The model under review builds one solid part; all positions refer to its coordinate system, in mm. A direction names the side the tool comes from. Coordinates: 2 decimals unless noted, no trailing zeros. Write each loop counter-clockwise with the first axis right and the second up, starting at its lowest first coordinate (ties: lowest second). Pieces come first, ordered by that corner, then holes. Notation, with made-up numbers: (58, 47) - (70, 47) arc R21 cw to (70, 86) - close; hole circle Ø5 at (13.25, 28.5). An arc over 180 degrees is marked (long way). Put each result on its own line as item: value. Start each with the question number.
Item 1: For pin 1 (2.5 mm diameter, centred on y = 47.5, z = -42.5, fed in from +X); pin 2 (1 mm diameter, centred on y = 2, z = -11.5, fed in from +X); pin 3 (12.5 mm diameter, centred on x = 39.41, y = 63.5, fed in from -Z); pin 4 (1.5 mm diameter, centred on y = 15, z = 37, fed in from +X), all flat-tipped, find the tip position at first contact; note any pin that passes through.
Item 2: Machinability: for faces 4 (the face through (-47, 2, 21.902)), 5 (the face through (17.18, 2, 13)), 6 (the face through (-47, 75, -0.323)), 7 (the face through (-4.796, 28.121, 67.961)), 8 (the face through (-38, 73.025, -12)), which of the approach directions +Z, -Z, +X, -X, +Y, -Y give a long, thin tool a straight path to every point of the face, cutting with its end or side? Answer none if there is none.
Item 3: Consider section D-D on y = 68.5. Give the boundary of the cut face in (x, z), then the cut area to 3 significant figures.
Item 4: Consider section B-B on x = 1. State how many separate pieces and enclosed holes the cut face has, then the cut area to 3 significant figures.
Item 5: Consider section A-A on z = 6.5. Give the boundary of the cut face in (x, y) (1 decimal).
Item 6: To check wall thickness, follow L1, parallel to Z at x = 34, y = 69.5; L2, parallel to Y at x = 6, z = -34 (3 decimals); L3, parallel to X at y = 24.5, z = 58. State the ranges of each line that lie inside material, in increasing order. Write a range as [from, to].
Item 7: Consider section C-C on z = -20.5. Give the boundary of the cut face in (x, y) (1 decimal).
Item 8: Mouldability with a two-part tool opening along Y and no side actions: class faces 1 (the face through (43.886, 32.194, 67.917)), 2 (the face through (4.55, 1.565, 45.713)), 3 (the face through (-36, 12.7, 68)) as pulls with the +Y half, pulls with the -Y half, needs draft (parallel to the pull), parting line crosses it, or undercut.
```python
from build123d import *

# Parameters (mm, degrees)
SKETCH1_W               = 152.4
SKETCH1_H               = 114.3
BOSS_EXTRUDE1_DEPTH     = 76.2
CUT_EXTRUDE1_DEPTH      = 142.677746119
CUT_EXTRUDE1_DEPTH_BACK = 142.677746119
SKETCH5_W               = 38.1
SKETCH5_H               = 107.95
CUT_EXTRUDE4_DEPTH      = 142.677746119
CUT_EXTRUDE5_DEPTH      = 169.235334824
CUT_EXTRUDE5_DEPTH_BACK = 169.235334824
SKETCH6_R               = 7.9375
CUT_EXTRUDE6_START      = -114.3
SKETCH8_W               = 107.95
SKETCH8_H               = 69.85
CUT_EXTRUDE6_DEPTH      = 111.125
SKETCH9_R               = 1.5875
CUT_EXTRUDE7_DEPTH      = 3.175
SKETCH10_W              = 88.9
SKETCH10_H              = 19.05
CUT_EXTRUDE8_DEPTH      = 5.715
CUT_EXTRUDE9_DEPTH      = 169.235334824
SKETCH13_W              = 76.2
SKETCH13_H              = 25.4
CUT_EXTRUDE10_DEPTH     = 5.715


with BuildPart() as part:
    # Sketch1 → Boss-Extrude1 (new body)
    with BuildSketch(Plane(origin=(0, 0, 0), x_dir=(1, 0, 0), z_dir=(0, 1, 0))):
        with Locations((-20.919503106, -12.376583851)):
            Rectangle(SKETCH1_W, SKETCH1_H)
    extrude(amount=BOSS_EXTRUDE1_DEPTH)

    # Sketch3 → Cut-Extrude1 (cut, two sides: drawn at the far end of the back side and taken through both)
    with BuildSketch(Plane.XY.offset(-CUT_EXTRUDE1_DEPTH_BACK)):
        Polygon((55.280496894, 63.5), (32.168387019, 0), (55.280496894, 0), align=None)
    extrude(amount=CUT_EXTRUDE1_DEPTH + CUT_EXTRUDE1_DEPTH_BACK, mode=Mode.SUBTRACT)

    # Sketch5 → Cut-Extrude4 (cut, through all)
    with BuildSketch(Plane(origin=(0, 0, 0), x_dir=(1, 0, 0), z_dir=(0, 1, 0))):
        with Locations((36.230496894, -12.376583851)):
            Rectangle(SKETCH5_W, SKETCH5_H)
    extrude(amount=CUT_EXTRUDE4_DEPTH, mode=Mode.SUBTRACT)

    # Sketch6 → Cut-Extrude5 (cut, two sides: drawn at the far end of the back side and taken through both)
    with BuildSketch(Plane.XY.offset(69.526583851).offset(-CUT_EXTRUDE5_DEPTH_BACK)):
        with Locations((39.405496894, 63.5)):
            Circle(SKETCH6_R)
    extrude(amount=CUT_EXTRUDE5_DEPTH + CUT_EXTRUDE5_DEPTH_BACK, mode=Mode.SUBTRACT)

    # Sketch8 → Cut-Extrude6 (cut)
    with BuildSketch(Plane.ZY.offset(97.119503106).offset(CUT_EXTRUDE6_START)):
        with Locations((12.376583851, 38.1)):
            Rectangle(SKETCH8_W, SKETCH8_H)
    extrude(amount=CUT_EXTRUDE6_DEPTH, mode=Mode.SUBTRACT)

    # Sketch9 → Cut-Extrude7 (cut)
    with BuildSketch(Plane.XZ):
        with Locations(Location((4.480496894, 44.126583851, 0), (0, 0, 270))):
            Circle(SKETCH9_R)
        with Locations(Location((-9.489503106, 44.126583851, 0), (0, 0, 270))):
            Circle(SKETCH9_R)
    extrude(amount=-CUT_EXTRUDE7_DEPTH, mode=Mode.SUBTRACT)

    # Sketch10 → Cut-Extrude8 (cut)
    with BuildSketch(Plane.XZ):
        with Locations((-46.319503106, 12.376583851)):
            Rectangle(SKETCH10_W, SKETCH10_H)
    extrude(amount=-CUT_EXTRUDE8_DEPTH, mode=Mode.SUBTRACT)

    # Sketch12 → Cut-Extrude9 (cut, through all)
    with BuildSketch(Plane.XY.offset(69.526583851)):
        Polygon((-73.343348256, 63.5), (2.929342045, 63.5), (-35.207003106, 43.816725084), align=None)
        Polygon((-84.419503106, 57.783274916), (-84.419503106, 18.416725084), (-46.283157955, 38.1), align=None)
        Polygon((-73.343348256, 12.7), (2.929342045, 12.7), (-35.207003106, 32.383274916), align=None)
        Polygon((14.005496894, 57.783274916), (14.005496894, 18.416725084), (-24.130848256, 38.1), align=None)
    extrude(amount=-CUT_EXTRUDE9_DEPTH, mode=Mode.SUBTRACT)

    # Sketch13 → Cut-Extrude10 (cut)
    with BuildSketch(Plane(origin=(0, 76.2, 0), x_dir=(1, 0, 0), z_dir=(0, 1, 0))):
        with Locations((-46.319503106, -12.376583851)):
            Rectangle(SKETCH13_W, SKETCH13_H)
    extrude(amount=-CUT_EXTRUDE10_DEPTH, mode=Mode.SUBTRACT)


solid = part.part
```
Report:
1. pin 1: x = 49.91
1. pin 2: x = 17.18
1. pin 3: through
1. pin 4: x = -93.94
2. face 4: -Y
2. face 5: +X, +Y, -Y
2. face 6: +Y
2. face 7: +Z, -Z
2. face 8: +X
3. outline: (-97.12, -44.77) - (33.24, -44.77) - (33.24, -41.6) - (-93.94, -41.6) - (-93.94, 66.35) - (33.24, 66.35) - (33.24, 69.53) - (-97.12, 69.53) - close; (45.57, -44.77) - (55.28, -44.77) - (55.28, -41.6) - (45.57, -41.6) - close; (45.57, 66.35) - (55.28, 66.35) - (55.28, 69.53) - (45.57, 69.53) - close
3. area: 1,230 mm²
4. separate pieces: 6
4. enclosed holes: 0
4. area: 992 mm²
5. outline: (-97.1, 0) - (-90.8, 0) - (-90.8, 3.2) - (-93.9, 3.2) - (-93.9, 73) - (-84.4, 73) - (-84.4, 76.2) - (-97.1, 76.2) - close; (-8.2, 73) - (17.2, 73) - (17.2, 76.2) - (-8.2, 76.2) - close; (-1.9, 0) - (17.2, 0) - (17.2, 3.2) - (-1.9, 3.2) - close
6. L1: [-44.77, -41.6], [66.35, 69.53]
6. L2: [0, 3.175], [73.025, 76.2]
6. L3: [-97.12, -93.94]
7. outline: (-97.1, 0) - (17.2, 0) - (17.2, 3.2) - (-93.9, 3.2) - (-93.9, 73) - (17.2, 73) - (17.2, 76.2) - (-97.1, 76.2) - close
8. face 1: pulls with the -Y half
8. face 2: needs draft
8. face 3: undercut
